Work out the finished part from the listing and answer in its coordinate system (mm). Face numbers are marked on the shaded views. A direction names the side the tool comes from. Round coordinates to 2 decimals unless told otherwise and drop trailing zeros. Write each loop counter-clockwise with the first axis right and the second up, starting at its lowest first coordinate (ties: lowest second). Pieces come first, ordered by that corner, then holes. Notation, with made-up numbers: M -14,1 L 7,1 A19 ccw 7,15 Z; hole C 26.5,38 d2. An arc over 180 degrees is marked long. One line per item, written item: value. Start each with the question number.
Q1. Find section D-D (x = 52.5). Write down the section's boundary in (y, z), and give its area (3 significant figures).
Q2. Find section A-A (x = 36). Write down the section's boundary in (y, z).
Q3. Find section B-B (y = 42.5). Write down the section's boundary in (x, z), and give its area (3 significant figures).
Q4. Consider probe 1 along X at (y, z) = (34, -11); probe 2 along Y at (x, z) = (-17.5, 29.5); probe 3 along Y at (x, z) = (50, -18.5). Determine where each line is inside the solid, lowest interval first.
Q5. Given pin 1 Ø11 at (x, y) = (75, -39.5) entering from +Z; pin 2 Ø8 at (x, z) = (87, 1.5) entering from +Y; pin 3 Ø12 at (x, z) = (21, 41.5) entering from +Y, each flat-ended and moving along its own axis, determine where each tip first touches the part or whether it passes through.
Q6. Find section C-C (z = -31). Write down the section's boundary in (x, y), and give its area (3 significant figures).
Q7. A tool of negligible diameter and unlimited length cuts with its end or side. For the marked faces 1 and 2, from which of +Z, -Z, +X, -X, +Y, -Y can it reach the whole face along a straight path? Write none if from no direction.
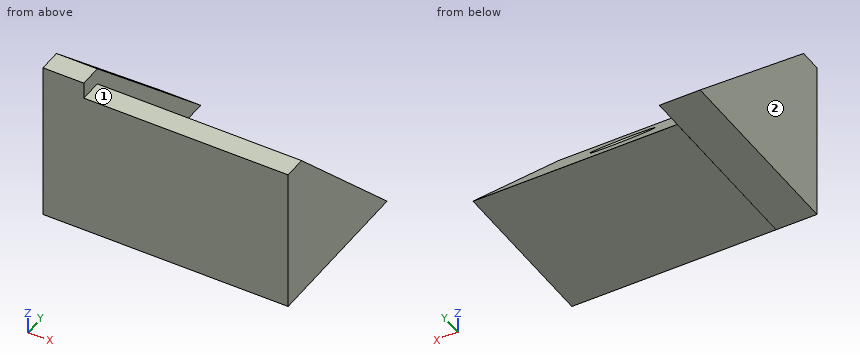
from build123d import *

# Parameters (mm, degrees)
F0_W     = 103.4859903157
F0_H     = 90.8377021551
F1_DEPTH = 127
F3_DEPTH = 127.001
F4_R     = 18.7473468239
F5_DEPTH = 25.4
F7_DEPTH = 127.001
F9_DEPTH = 25.4


with BuildPart() as f1:
    # F0 (on Right) → F1 (new body)
    with BuildSketch(Plane.YZ):
        with Locations((2.6829708368, 1.6289465129)):
            Rectangle(F0_W, F0_H)
    extrude(amount=F1_DEPTH)

    # F2 (on face) → F3 (cut, through all)
    with BuildSketch(Plane.YZ.offset(127)):
        Polygon((62.4748729169, 57.3963969946), (-45.2272109687, 71.7694461346), (64.1996413469, -25.7756765932), align=None)
    extrude(amount=-F3_DEPTH, mode=Mode.SUBTRACT)

    # F4 (on face) → F5 (cut)
    with BuildSketch(Plane(origin=(0, 15.6232196657, 17.5262453236), x_dir=(1, 0, 0), z_dir=(0, 0.6654180184, 0.7464709377))):
        with Locations((63.312150538, 0)):
            Circle(F4_R)
    extrude(amount=-F5_DEPTH, mode=Mode.SUBTRACT)

    # F6 (on face) → F7 (cut, through all)
    with BuildSketch(Plane(origin=(0, 0, 0), x_dir=(0, -1, 0), z_dir=(-1, 0, 0))):
        Polygon((-58.8337033987, -48.1976419687), (43.6940863729, 55.8632686734), (45.8021350205, 72.5360140204), (-54.4259659946, 13.5106705129), align=None)
    extrude(amount=-F7_DEPTH, mode=Mode.SUBTRACT)

    # F8 (on face) → F9 (join)
    with BuildSketch(Plane(origin=(0, 0, 0), x_dir=(0, -1, 0), z_dir=(-1, 0, 0))):
        Polygon((49.0600243211, -43.7899045646), (49.0600243211, 47.0477975905), (49.0600243211, 57.3963969946), (35.0084929031, 57.3963969946), (-73.2067525387, -43.7239946857), align=None)
    extrude(amount=F9_DEPTH)


solid = f1.part
The answers:
1. outline: M -49.06,-43.79 L 54.43,-43.79 L 54.43,-43.72 L 16.16,-4.89 L 10.15,-11.63 L -12.71,8.76 L -5.38,16.98 L -35.01,47.05 L -49.06,47.05 Z
1. area: 5,030 mm2
2. outline: M -49.06,-43.79 L 54.43,-43.79 L 54.43,-43.72 L -35.01,47.05 L -49.06,47.05 Z
3. outline: M -25.4,-43.74 L 0,-43.74 L 0,-43.79 L 127,-43.79 L 127,-31.62 L 0,-31.62 L 0,-15.03 L -25.4,-15.03 Z
3. area: 2,270 mm2
4. probe 1: -25.4 to 0
4. probe 2: -49.06 to -5.15
4. probe 3: -49.06 to 29.57
5. pin 1: z = 47.05
5. pin 2: y = 13.81
5. pin 3: y = -23.63
6. outline: M -25.4,-49.06 L 127,-49.06 L 127,41.89 L 0,41.89 L 0,59.59 L -25.4,59.59 Z
6. area: 14,300 mm2
7. face 1: +Z, +X, +Y, -Y
7. face 2: +Z, -Z, -X, +Y, -Y
